Model file for the job. Use its own axes, mm. A direction names the side the tool comes from. Round coordinates to 2 decimals unless told otherwise and drop trailing zeros. Order: outer loops, then holes, each group sorted by start corner. A loop starts at its lowest first (then second) coordinate and runs counter-clockwise, first axis right, second up. Notation, with made-up numbers: (8, -35) - (32, -35) arc R15 ccw to (32, -10) - close; hole circle Ø4 at (-9.5, 56). An arc over 180 degrees is marked (long way). Use one line per item in the form item = value.
from build123d import *

# Parameters (mm, degrees)
SKETCH1_W           = 88.9
SKETCH1_H           = 19.05
BOSS_EXTRUDE1_DEPTH = 3.175
SKETCH2_W           = 3.302
SKETCH2_H           = 3.302
CUT_EXTRUDE1_DEPTH  = 46.5698228
SKETCH3_W           = 5.08
SKETCH3_H           = 3.175
SKETCH3_W_2         = 88.9
BOSS_EXTRUDE2_DEPTH = 3.175


with BuildPart() as part:
    # Sketch1 → Boss-Extrude1 (new body)
    with BuildSketch(Plane(origin=(0, 0, 0), x_dir=(1, 0, 0), z_dir=(0, 1, 0))):
        Rectangle(SKETCH1_W, SKETCH1_H)
    extrude(amount=BOSS_EXTRUDE1_DEPTH)

    # Sketch2 → Cut-Extrude1 (cut, through all)
    with BuildSketch(Plane(origin=(0, 3.175, 0), x_dir=(1, 0, 0), z_dir=(0, 1, 0))):
        with Locations((-42.799, 4.7625)):
            Rectangle(SKETCH2_W, SKETCH2_H)
        with Locations((-42.799, -1.5875)):
            Rectangle(SKETCH2_W, SKETCH2_H)
        with Locations((-42.799, -7.9375)):
            Rectangle(SKETCH2_W, SKETCH2_H)
        with Locations((42.799, -7.9375)):
            Rectangle(SKETCH2_W, SKETCH2_H)
        with Locations((42.799, -1.5875)):
            Rectangle(SKETCH2_W, SKETCH2_H)
        with Locations((42.799, 4.7625)):
            Rectangle(SKETCH2_W, SKETCH2_H)
    extrude(amount=-CUT_EXTRUDE1_DEPTH, mode=Mode.SUBTRACT)

    # Sketch3 → Boss-Extrude2 (add)
    with BuildSketch(Plane(origin=(0, 0, 0), x_dir=(1, 0, 0), z_dir=(0, 1, 0))):
        with Locations((-25.4, -11.1125)):
            Rectangle(SKETCH3_W, SKETCH3_H)
        with Locations((-15.24, -11.1125)):
            Rectangle(SKETCH3_W, SKETCH3_H)
        with Locations((0, 11.1125)):
            Rectangle(SKETCH3_W_2, SKETCH3_H)
        with Locations((-5.08, -11.1125)):
            Rectangle(SKETCH3_W, SKETCH3_H)
        with Locations((5.08, -11.1125)):
            Rectangle(SKETCH3_W, SKETCH3_H)
        with Locations((15.24, -11.1125)):
            Rectangle(SKETCH3_W, SKETCH3_H)
        with Locations((25.4, -11.1125)):
            Rectangle(SKETCH3_W, SKETCH3_H)
    extrude(amount=BOSS_EXTRUDE2_DEPTH)


solid = part.part
(1) Slice it at C-C on z = -4.75. Give the cut face in (x, y) (3 decimals), then the cut area to 3 significant figures.
Report:
outline = (-41.148, 0) - (41.148, 0) - (41.148, 3.175) - (-41.148, 3.175) - close
area = 261 mm2
(2) Slice it at B-B on x = 37. Give the cut face in (y, z) (3 decimals).
Report:
outline = (0, -12.7) - (3.175, -12.7) - (3.175, 9.525) - (0, 9.525) - close
(3) Pin check, flat tips, straight feed: pin 1 (1 mm diameter, centred on x = 31.5, y = 1.5, fed in from +Z) (3 decimals); pin 2 (1 mm diameter, centred on x = 42, y = 2, fed in from +Z); pin 3 (1.6 mm diameter, centred on y = 2.5, z = 11.5, fed in from +X). Stop position of each tip, or through.
Report:
pin_1 = 9.525
pin_2 = 6.29
pin_3 = 27.94
(4) Slice it at A-A on z = 10.75. Give the cut face in (x, y) (3 decimals), then the cut area to 3 significant figures.
Report:
outline = (-27.94, 0) - (-22.86, 0) - (-22.86, 3.175) - (-27.94, 3.175) - close; (-17.78, 0) - (-12.7, 0) - (-12.7, 3.175) - (-17.78, 3.175) - close; (-7.62, 0) - (-2.54, 0) - (-2.54, 3.175) - (-7.62, 3.175) - close; (2.54, 0) - (7.62, 0) - (7.62, 3.175) - (2.54, 3.175) - close; (12.7, 0) - (17.78, 0) - (17.78, 3.175) - (12.7, 3.175) - close; (22.86, 0) - (27.94, 0) - (27.94, 3.175) - (22.86, 3.175) - close
area = 96.8 mm2
(5) Pull direction X, two halves, no side cores. Call faces 5 (the face through (7.62, 2, 11)), 6 (the face through (43, 2, -6.414)), 7 (the face through (-27.94, 2, 11)): released by +X, released by -X, zero draft, split by the parting line, or undercut.
Report:
face_5 = undercut
face_6 = zero draft
face_7 = released by -X
(6) Tool access for faces 1 (the face through (43, 2, 3.238)), 2 (the face through (41.148, 2, 8)), 3 (the face through (-2.54, 2, 11)), 4 (the face through (-43, 2, 3.238)): list every direction of +Z, -Z, +X, -X, +Y, -Y with a clear straight run to the whole face (end or side of a thin tool).
Report:
face_1 = +X, +Y, -Y
face_2 = +Z, +X, +Y, -Y
face_3 = +Z, +Y, -Y
face_4 = -X, +Y, -Y
(7) Probe probe 1 along Z at (x, y) = (-20, 1.1) (3 decimals); probe 2 along X at (y, z) = (0.6, 8.5). List the from-to ranges inside material, lowest first. Write a range as [from, to].
Report:
probe_1 = [-12.7, 9.525]
probe_2 = [-41.15, 41.15]
